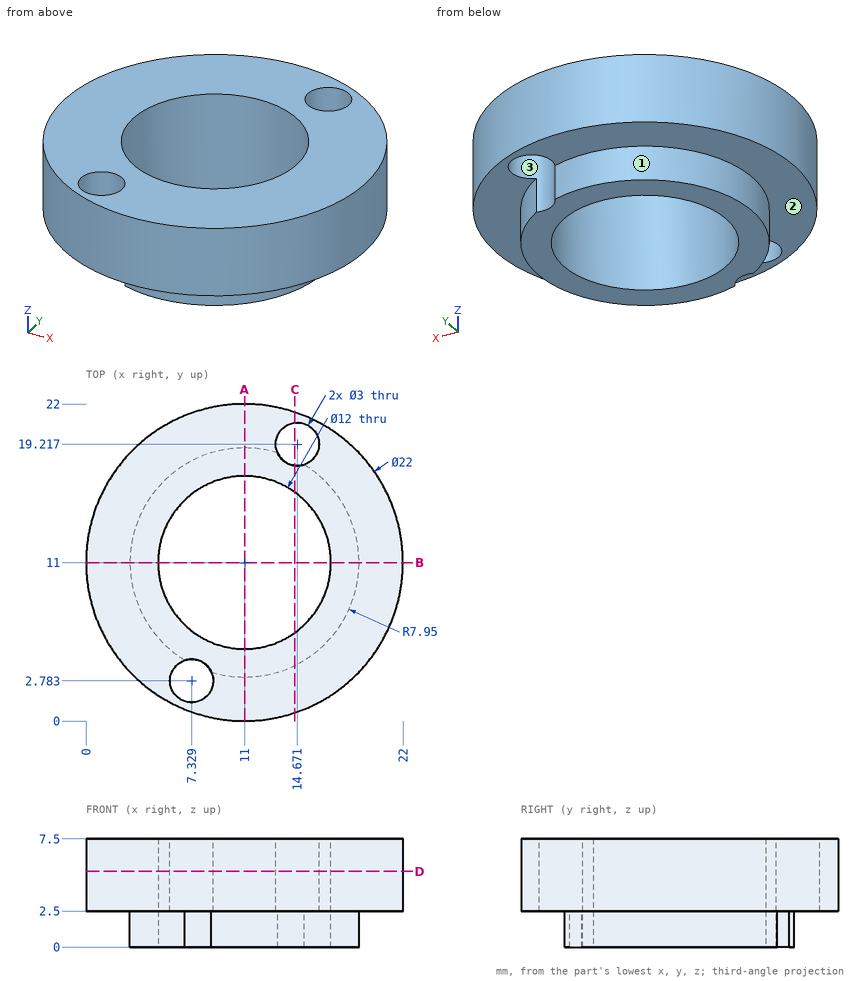
For this review, use the dimensioned drawing (mm, ordinates from the lowest corner) and the shaded views. Give positions to 0.01 mm unless a question says otherwise; leave off trailing zeros. Loops run counter-clockwise (first coordinate to the right, second up) from the corner with the lowest first, then second, coordinate; pieces in that order, holes last. Notation, with made-up numbers: (-32.75, 0) -> (-20.75, 0) arc R13 ccw to (-20.75, 9) -> close; hole circle Ø4 at (21.5, 6). An arc over 180 degrees is marked (long way). Use CSV: the item, a comma, the result in double quotes.
1. To check wall thickness, follow probe 1 along Y at (x, z) = (8, 6) (1 decimal); probe 2 along Y at (x, z) = (14.25, 4); probe 3 along X at (y, z) = (10.75, 4.5) (1 decimal). State the ranges of each line that lie inside material, in increasing order. Write a range as from..to.
Result:
probe 1,"y = 0.4..1.4, 4.1..5.8, 16.2..21.6"
probe 2,"y = 0.49..5.96, 16.04..17.78, 20.66..21.51"
probe 3,"x = 0..5, 17..22"
2. For P1, Ø1.5, axis at x = 19, y = 16.5, coming from the -Z side; P2, Ø2, axis at y = 8, z = 5, coming from the -X side, all flat-tipped, find the tip position at first contact; note any pin that passes through.
Result:
P1,"stops at z = 2.5"
P2,"stops at x = 0.18"
3. Consider section C-C, the plane x = 14.5. Write out the cut boundary in (y, z).
Result:
outline,"(0.57, 2.5) -> (3.86, 2.5) -> (3.86, 0) -> (6.13, 0) -> (6.13, 7.5) -> (0.57, 7.5) -> close; (15.87, 0) -> (17.73, 0) -> (17.73, 7.5) -> (15.87, 7.5) -> close; (20.71, 2.5) -> (21.43, 2.5) -> (21.43, 7.5) -> (20.71, 7.5) -> close"
4. Consider section D-D, the plane z = 5.25. Write out the cut boundary in (x, y).
Result:
outline,"circle Ø22 at (11, 11); hole circle Ø12 at (11, 11); hole circle Ø3 at (7.33, 2.78); hole circle Ø3 at (14.67, 19.22)"
5. The part is to be moulded in two halves that separate along Y. For the marked faces 1, 2 and 3, say which applies: +Y half, -Y half, draft (parallel to the pull), parting line (faces both ways), or undercut.
Result:
face 1,"parting line"
face 2,"draft"
face 3,"undercut"
6. Consider section A-A, the plane x = 11. Write out the cut boundary in (y, z).
Result:
outline,"(0, 2.5) -> (3.05, 2.5) -> (3.05, 0) -> (5, 0) -> (5, 7.5) -> (0, 7.5) -> close; (17, 0) -> (18.95, 0) -> (18.95, 2.5) -> (22, 2.5) -> (22, 7.5) -> (17, 7.5) -> close"
